from build123d import *

# Parameters (mm, degrees)
SKETCH1_W           = 60
SKETCH1_H           = 50
SKETCH1_R           = 5
SKETCH1_R_2         = 1.5
BOSS_EXTRUDE1_DEPTH = 4
CUT_EXTRUDE1_DEPTH  = 5


with BuildPart() as part:
    # Sketch1 → Boss-Extrude1 (new body)
    with BuildSketch(Plane.XY):
        Rectangle(SKETCH1_W, SKETCH1_H)
        Circle(SKETCH1_R, mode=Mode.SUBTRACT)
        with Locations((-8.5, 0)):
            Circle(SKETCH1_R_2, mode=Mode.SUBTRACT)
        with Locations((8.5, 0)):
            Circle(SKETCH1_R_2, mode=Mode.SUBTRACT)
    extrude(amount=BOSS_EXTRUDE1_DEPTH)

    # Sketch2 → Cut-Extrude1 (cut, through all)
    with BuildSketch(Plane.XY.offset(4)):
        Polygon((-17.5, -5), (-22.5, -5), (-22.5, -10.5), (-25, -10.5), (-25, -15.5), (-22.5, -15.5), (-22.5, -25), (-17.5, -25), (-17.5, -15.5), (-15, -15.5), (-15, -10.5), (-17.5, -10.5), align=None)
        Polygon((22.5, -5), (17.5, -5), (17.5, -10.5), (15, -10.5), (15, -15.5), (17.5, -15.5), (17.5, -25), (22.5, -25), (22.5, -15.5), (25, -15.5), (25, -10.5), (22.5, -10.5), align=None)
    extrude(amount=-CUT_EXTRUDE1_DEPTH, mode=Mode.SUBTRACT)


solid = part.part
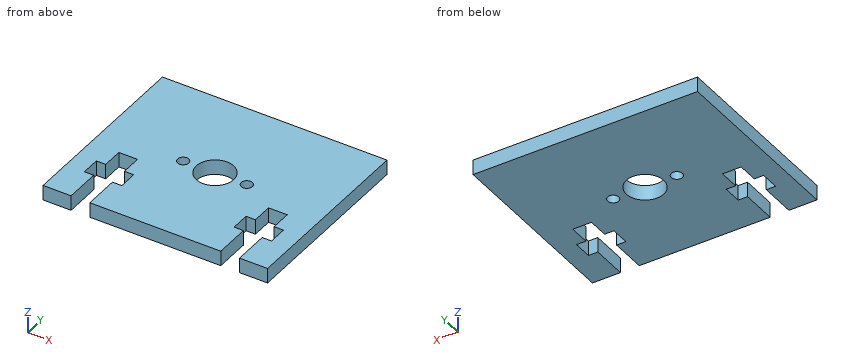
Read the model definition and answer for the solid it produces. Units are mm, in the model's axes. Coordinates: 2 decimals unless noted, no trailing zeros. Write each loop counter-clockwise with the first axis right and the second up, starting at its lowest first coordinate (ties: lowest second). Pieces come first, ordered by that corner, then holes. Notation, with made-up numbers: M 7,-9 L 51,-9 A37 ccw 51,29 Z; hole C 34,-32 d5. An arc over 180 degrees is marked long. Use a Markdown table: item, result.
Q1. The part is cut by section A-A, the plane y = 4. Write down the section's boundary in (x, z).
Answer block:
| item | result |
|---|---|
| outline | M -30,0 L -3,0 L -3,4 L -30,4 Z; M 3,0 L 30,0 L 30,4 L 3,4 Z |
Q2. Straight lines are drawn through the part: L1, parallel to X at y = -7, z = 2.3; L2, parallel to Y at x = -8.5, z = 1.75; L3, parallel to Y at x = 0, z = 1.3. For each, find the intervals that lie inside material, in ascending order. Write a range as [from, to].
Answer block:
| item | result |
|---|---|
| L1 | x = [-30, -22.5], [-17.5, 17.5], [22.5, 30] |
| L2 | y = [-25, -1.5], [1.5, 25] |
| L3 | y = [-25, -5], [5, 25] |
Q3. The part is cut by section C-C, the plane y = -7.5. Write down the section's boundary in (x, z).
Answer block:
| item | result |
|---|---|
| outline | M -30,0 L -22.5,0 L -22.5,4 L -30,4 Z; M -17.5,0 L 17.5,0 L 17.5,4 L -17.5,4 Z; M 22.5,0 L 30,0 L 30,4 L 22.5,4 Z |
Q4. The part is cut by section B-B, the plane x = 8.5. Write down the section's boundary in (y, z).
Answer block:
| item | result |
|---|---|
| outline | M -25,0 L -1.5,0 L -1.5,4 L -25,4 Z; M 1.5,0 L 25,0 L 25,4 L 1.5,4 Z |
Q5. The part is cut by section D-D, the plane z = 2.25. Give the number of separate pieces and of enclosed holes in the cut face, then the cut area to 3 significant figures.
Answer block:
| item | result |
|---|---|
| separate pieces | 1 |
| enclosed holes | 3 |
| area | 2,660 mm2 |
